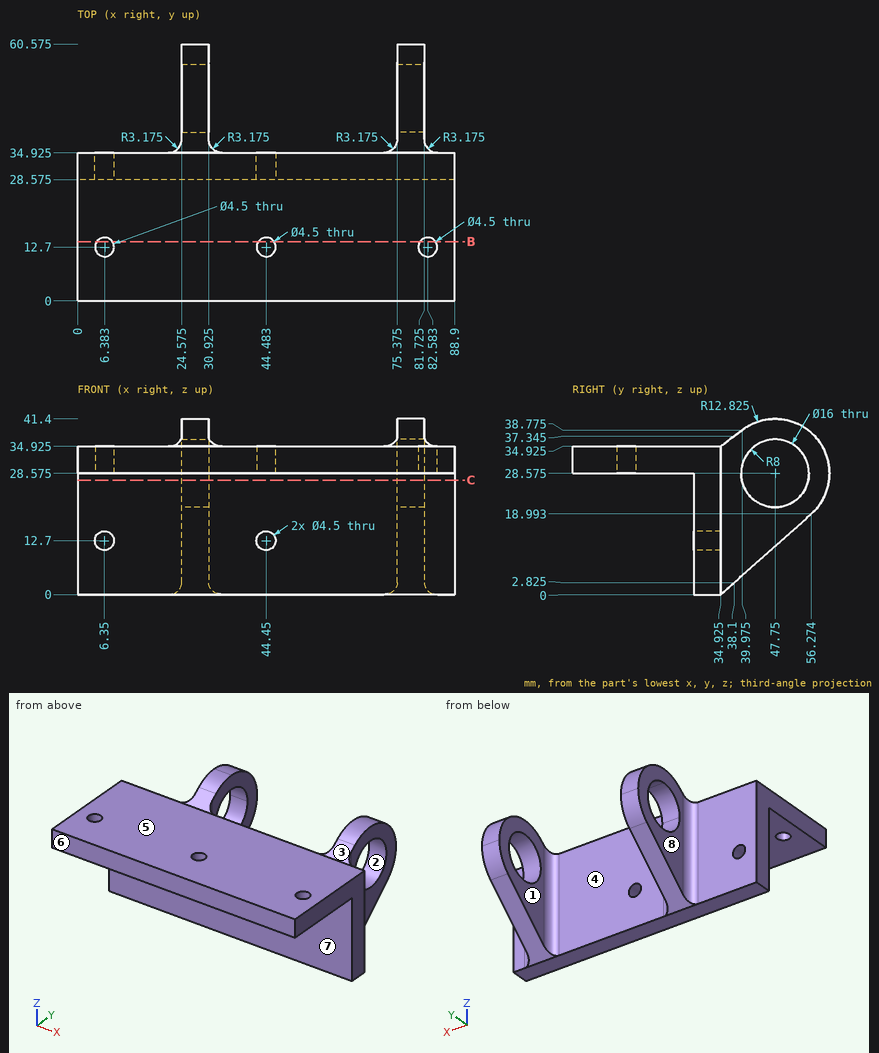
Answer from the drawing. Dimensions are ordinates in mm from the lowest x, y and z of the part. A direction names the side the tool comes from. Give positions to 0.01 mm unless a question says otherwise; leave off trailing zeros. Write each loop counter-clockwise with the first axis right and the second up, starting at its lowest first coordinate (ties: lowest second). Pieces come first, ordered by that corner, then holes. Notation, with made-up numbers: (68.5, 53) -> (98.5, 53) arc R20 ccw to (98.5, 57) -> close; hole circle Ø6 at (33.25, 61). An arc over 180 degrees is marked (long way). One line per question, with ' | ' between items. Start each with the question number.
1. Section C-C (z = 27) is taken. State how many separate pieces and enclosed holes the cut face has.
2. Find the intervals of material crossed by probe 1 along X at (y, z) = (56, 37) (1 decimal); probe 2 along X at (y, z) = (33, 12); probe 3 along Y at (x, z) = (49.5, 19.5) (1 decimal), in increasing order.
3. For a pull along Z with two mould halves and no side action, classify the marked faces 1, 2 and 3 as pulls with the +Z half, pulls with the -Z half, needs draft (parallel to the pull), parting line crosses it, or undercut.
4. Given pin 1 Ø9.5 at (y, z) = (47.75, 28.575) entering from +X; pin 2 Ø3 at (x, z) = (87.5, 17) entering from +Y (3 decimals); pin 3 Ø1.5 at (x, z) = (35, 22) entering from -Y (3 decimals); pin 4 Ø18 at (y, z) = (52, 31.5) entering from +X (3 decimals), each flat-ended and moving along its own axis, determine where each tip first touches the part or whether it passes through.
5. For the marked faces 4, 5, 6, 7 and 8, determine the directions among +Z, -Z, +X, -X, +Y, -Y from which every point of the face is accessible in a straight line to the end or side of a thin tool.
6. Section B-B (y = 14) is taken. Determine the outline of the cut face in (x, z) (1 decimal).
Response values:
1) separate pieces: 3 | enclosed holes: 0
2) probe 1: 24.6 to 30.9, 75.4 to 81.7 | probe 2: 0 to 4.21, 8.49 to 42.31, 46.59 to 88.9 | probe 3: 28.6 to 34.9
3) face 1: needs draft | face 2: undercut | face 3: pulls with the +Z half
4) pin 1: through | pin 2: y = 34.925 | pin 3: y = 28.575 | pin 4: x = 81.725
5) face 4: +Z, -Z, +Y | face 5: +Z, +X, -X, -Y | face 6: +Z, -Z, +X, -X, -Y | face 7: -Z, +X, -X, -Y | face 8: +Z, -Z, -X, +Y
6) outline: (0, 28.6) -> (4.5, 28.6) -> (4.5, 34.9) -> (0, 34.9) -> close; (8.2, 28.6) -> (42.6, 28.6) -> (42.6, 34.9) -> (8.2, 34.9) -> close; (46.3, 28.6) -> (80.7, 28.6) -> (80.7, 34.9) -> (46.3, 34.9) -> close; (84.4, 28.6) -> (88.9, 28.6) -> (88.9, 34.9) -> (84.4, 34.9) -> close
